Check sheet for the modelled part. Datum: model origin and axes. Units: mm. Face numbers are marked on the shaded views. A direction names the side the tool comes from. Round coordinates to 2 decimals unless told otherwise and drop trailing zeros. Write each loop counter-clockwise with the first axis right and the second up, starting at its lowest first coordinate (ties: lowest second). Pieces come first, ordered by that corner, then holes.
Item 1: Material ranges on line 1 (Y direction, x = 34, z = 12); line 2 (Y direction, x = -77, z = -19.5); line 3 (Z direction, x = 7.5, y = -14.5), recorded low to high.
Item 2: Cross-section at C-C on x = -7.5. Enter the section's corners in (y, z).
Item 3: Tool access check on the marked faces 4, 5, 6 and 7. Record the directions out of +Z, -Z, +X, -X, +Y, -Y that give a thin tool (end or side, any length) a straight path to the whole face; none if there is none.
Item 4: Release check for a two-part mould opening along Z. For the marked faces 1, 2 and 3 record: +Z half, -Z half, draft (parallel to the pull), parting line (faces both ways), or undercut.
Item 5: Cross-section at B-B on z = 31. Enter the section's corners in (x, y), plus the area to 3 significant figures.
Item 6: Go/stop test with flat-tipped pins: pin 1 Ø20.5 at (y, z) = (-137, 15) entering from +X; pin 2 Ø8 at (y, z) = (-42.5, 0.5) entering from -X; pin 3 Ø10 at (x, z) = (-38.5, 25) entering from +Y; pin 4 Ø25 at (x, z) = (22.5, 20) entering from +Y. Record where each tip stops, or that it passes through.
Item 7: Cross-section at D-D on x = 14. Enter the section's corners in (y, z), plus the area to 3 significant figures.
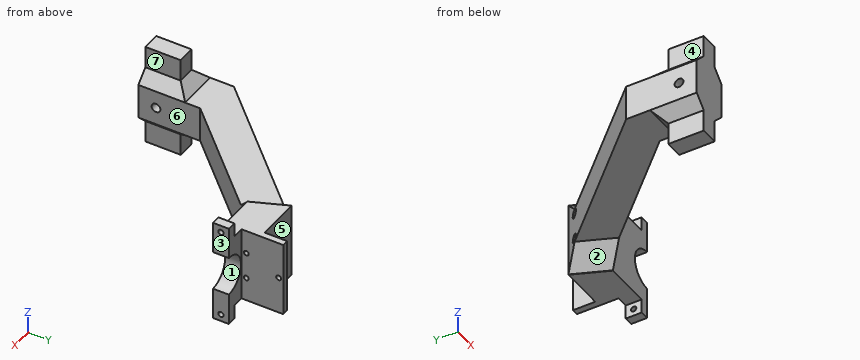
from build123d import *

# Parameters (mm, degrees)
BOSS_EXTRUDE1_DEPTH      = 25.4
BOSS_EXTRUDE4_DEPTH      = 24.13
BOSS_EXTRUDE4_DEPTH_BACK = 49.53
SKETCH7_W                = 12.7
SKETCH7_H                = 25.4
SKETCH8_R                = 3.175
CUT_EXTRUDE3_DEPTH       = 219.535967291
CHAMFER3_SIZE            = 8.255
BOSS_EXTRUDE5_DEPTH      = 14.224
BOSS_EXTRUDE5_DEPTH_BACK = 39.624
SKETCH9_R                = 14.224
CUT_EXTRUDE4_DEPTH       = 188.728167838
SKETCH11_W               = 14.732
SKETCH11_H               = 53.848
CUT_EXTRUDE5_DEPTH       = 13.97
CHAMFER5_SIZE            = 13.97
SKETCH18_W               = 6.35
SKETCH18_H               = 11.43
BOSS_EXTRUDE6_DEPTH      = 10.16
SKETCH19_W               = 6.35
SKETCH19_H               = 11.43
BOSS_EXTRUDE7_DEPTH      = 10.16
SKETCH20_R               = 1.905
CUT_EXTRUDE7_DEPTH       = 10.16
SKETCH21_W               = 4.572
SKETCH21_H               = 53.848
BOSS_EXTRUDE8_DEPTH      = 16.129
SKETCH22_R               = 1.778
CUT_EXTRUDE8_DEPTH       = 4.318
SKETCH23_R               = 2.794
CUT_EXTRUDE9_DEPTH       = 207.118456854


with BuildPart() as part:
    # Sketch2 → Boss-Extrude1 (new body)
    with BuildSketch(Plane.XY):
        Polygon((0, 0), (50.8, 0), (50.8, -25.4), (10.806439585, -25.4), (-68.58, -107.87941775), (-68.58, -152.4), (-97.79, -152.4), (-97.79, -101.6), align=None)
    extrude(amount=BOSS_EXTRUDE1_DEPTH)

    # Sketch7 → Boss-Extrude4 (add, two sides: drawn at the far end of the back side and taken through both)
    with BuildSketch(Plane.XY.offset(25.4).offset(-BOSS_EXTRUDE4_DEPTH_BACK)):
        with Locations((-83.185, -139.7)):
            Rectangle(SKETCH7_W, SKETCH7_H)
    extrude(amount=BOSS_EXTRUDE4_DEPTH + BOSS_EXTRUDE4_DEPTH_BACK)

    # Sketch8 → Cut-Extrude3 (cut, through all)
    with BuildSketch(Plane.ZY.offset(97.79)):
        with Locations((12.7, -139.7)):
            Circle(SKETCH8_R)
    extrude(amount=-CUT_EXTRUDE3_DEPTH, mode=Mode.SUBTRACT)

    # Chamfer3
    chamfer3_edges = [part.edges().sort_by_distance(p)[0] for p in [
        (-76.835, -139.7, 25.4),
        (-76.835, -139.7, 0),
        (-83.185, -127, 25.4),
        (-83.185, -127, 0),
        (-89.535, -139.7, 25.4),
        (-89.535, -139.7, 0),
    ]]
    chamfer(chamfer3_edges, length=CHAMFER3_SIZE - 0.0001)  # a hair under: the kernel refuses the full size

    # Sketch10 → Boss-Extrude5 (add, two sides: drawn at the far end of the back side and taken through both)
    with BuildSketch(Plane.XY.offset(25.4).offset(-BOSS_EXTRUDE5_DEPTH_BACK)):
        Polygon((0, 0), (10.806439585, -25.4), (50.8, -25.4), (50.8, 0), align=None)
    extrude(amount=BOSS_EXTRUDE5_DEPTH + BOSS_EXTRUDE5_DEPTH_BACK)

    # Sketch9 → Cut-Extrude4 (cut, through all)
    with BuildSketch(Plane(origin=(0, 0, 0), x_dir=(1, 0, 0), z_dir=(0, 1, 0))):
        with Locations((50.8, -12.7)):
            Circle(SKETCH9_R)
    extrude(amount=-CUT_EXTRUDE4_DEPTH, mode=Mode.SUBTRACT)

    # Sketch11 → Cut-Extrude5 (cut)
    with BuildSketch(Plane(origin=(0, 0, 0), x_dir=(1, 0, 0), z_dir=(0, 1, 0))):
        with Locations((43.434, -12.7)):
            Rectangle(SKETCH11_W, SKETCH11_H)
    extrude(amount=-CUT_EXTRUDE5_DEPTH, mode=Mode.SUBTRACT)

    # Chamfer5
    chamfer5_edges = [part.edges().sort_by_distance(p)[0] for p in [
        (5.403219792, -12.7, 0),
        (5.403219792, -12.7, 25.4),
    ]]
    chamfer(chamfer5_edges, length=CHAMFER5_SIZE)

    # Sketch18 → Boss-Extrude6 (add)
    with BuildSketch(Plane.XY.offset(39.624)):
        with Locations((47.625, -19.685)):
            Rectangle(SKETCH18_W, SKETCH18_H)
    extrude(amount=BOSS_EXTRUDE6_DEPTH)

    # Sketch19 → Boss-Extrude7 (add)
    with BuildSketch(Plane(origin=(0, 0, -14.224), x_dir=(-1, 0, 0), z_dir=(0, 0, -1))):
        with Locations((-47.625, -19.685)):
            Rectangle(SKETCH19_W, SKETCH19_H)
    extrude(amount=BOSS_EXTRUDE7_DEPTH)

    # Sketch20 → Cut-Extrude7 (cut)
    with BuildSketch(Plane(origin=(50.8, 0, 0), x_dir=(0, 0, -1), z_dir=(1, 0, 0))):
        with Locations((-44.704, -19.685)):
            Circle(SKETCH20_R)
        with Locations((19.304, -19.685)):
            Circle(SKETCH20_R)
    extrude(amount=-CUT_EXTRUDE7_DEPTH, mode=Mode.SUBTRACT)

    # Sketch21 → Boss-Extrude8 (add)
    with BuildSketch(Plane(origin=(0, 0, 0), x_dir=(1, 0, 0), z_dir=(0, 1, 0))):
        with Locations((33.782, -12.7)):
            Rectangle(SKETCH21_W, SKETCH21_H)
    extrude(amount=BOSS_EXTRUDE8_DEPTH)

    # Sketch22 → Cut-Extrude8 (cut)
    with BuildSketch(Plane(origin=(36.068, 0, 0), x_dir=(0, 0, -1), z_dir=(1, 0, 0))):
        with Locations((-12.7, 12.827)):
            Circle(SKETCH22_R)
        with Locations((-22.352, -10.4775)):
            Circle(SKETCH22_R)
        with Locations((-3.048, -10.4775)):
            Circle(SKETCH22_R)
    extrude(amount=-CUT_EXTRUDE8_DEPTH, mode=Mode.SUBTRACT)

    # Sketch23 → Cut-Extrude9 (cut, through all)
    with BuildSketch(Plane(origin=(31.75, 0, 0), x_dir=(0, 0, -1), z_dir=(1, 0, 0))):
        with Locations((-22.352, -10.4775)):
            Circle(SKETCH23_R)
        with Locations((-3.048, -10.4775)):
            Circle(SKETCH23_R)
    extrude(amount=-CUT_EXTRUDE9_DEPTH, mode=Mode.SUBTRACT)


solid = part.part
Response values:
1. line 1: y = -25.4 to 11.19, 14.46 to 16.13
1. line 2: y = -152.4 to -127
1. line 3: z = -14.22 to 39.62
2. outline: (-44.42, 0) - (-18.06, 0) - (-7.79, -4.02) - (-7.79, 2.28) arc R2.79 cw (long way) to (-7.79, 3.82) - (-7.79, 21.58) arc R2.79 cw (long way) to (-7.79, 23.12) - (-7.79, 29.42) - (-18.06, 25.4) - (-44.42, 25.4) - close
3. face 4: +Z, -X, +Y, -Y
3. face 5: +Z, -Z, -X, +Y
3. face 6: +Z, -Z, +X, -Y
3. face 7: +Z, +X, +Y, -Y
4. face 1: undercut
4. face 2: -Z half
4. face 3: draft
5. outline: (-92.19, -152.4) - (-74.18, -152.4) - (-74.18, -124.35) - (-92.19, -124.35) - close; (-6.31, -6.55) - (4.5, -31.95) - (10.81, -25.4) - (50.8, -25.4) - (50.8, -13.97) - (36.07, -13.97) - (36.07, 16.13) - (31.5, 16.13) - (31.5, 0) - (0, 0) - close
5. area: 1,760 mm2
6. pin 1: stops at x = -68.58
6. pin 2: stops at x = -44.76
6. pin 3: stops at y = -34.81
6. pin 4: stops at y = 16.13
7. outline: (-25.4, -14.22) - (0, -14.22) - (0, 39.62) - (-25.4, 39.62) - close; hole circle Ø5.59 at (-10.48, 3.05); hole circle Ø5.59 at (-10.48, 22.35)
7. area: 1,320 mm2
